The listing builds one solid part. Answer for the finished solid, in the listing's coordinates (mm). Face numbers are marked on the shaded views. A direction names the side the tool comes from. Round coordinates to 2 decimals unless told otherwise and drop trailing zeros. Loops run counter-clockwise (first coordinate to the right, second up) from the corner with the lowest first, then second, coordinate; pieces in that order, holes last. Notation, with made-up numbers: (-39.75, 51) - (-6.75, 51) arc R24 ccw to (-6.75, 71) - close; hole circle Ø3 at (34, 48). An arc over 180 degrees is marked (long way). One line per item, written item: value.
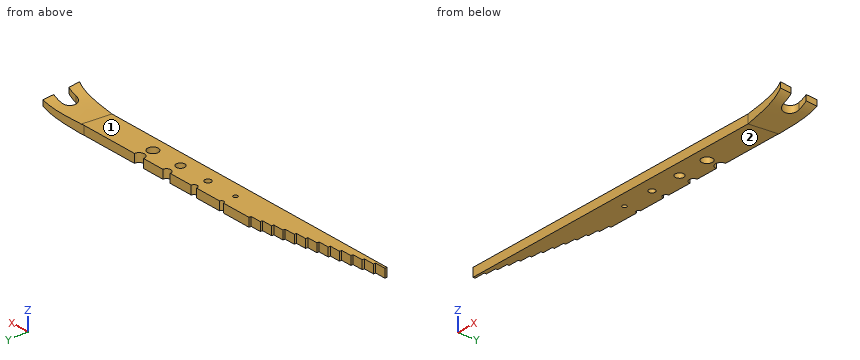
```python
from build123d import *

# Parameters (mm, degrees)
F0_R     = 1
F0_R_2   = 1.5
F0_R_3   = 2
F0_R_4   = 2.5
F1_DEPTH = 4
F3_DEPTH = 8
F5_DEPTH = 25


with BuildPart() as f1:
    # F0 (on Top) → F1 (new body)
    with BuildSketch(Plane.XY):
        with BuildLine():
            Line((-52.0707386732, -14.8954221606), (-52.0707386732, -15.8954221606))
            Line((-52.0707386732, -15.8954221606), (-57.0707386732, -15.8954221606))
            Line((-57.0707386732, -15.8954221606), (-57.0707386732, -16.8954221606))
            Line((-57.0707386732, -16.8954221606), (-62.0707386732, -16.8954221606))
            Line((-62.0707386732, -16.8954221606), (-62.0707386732, -17.8954221606))
            Line((-62.0707386732, -17.8954221606), (-67.0707386732, -17.8954221606))
            Line((-67.0707386732, -17.8954221606), (-67.0707386732, -18.8954221606))
            Line((-67.0707386732, -18.8954221606), (-72.0707386732, -18.8954221606))
            Line((-72.0707386732, -18.8954221606), (-72.0707386732, -19.8954221606))
            Line((-72.0707386732, -19.8954221606), (-77.0707386732, -19.8954221606))
            Line((-77.0707386732, -19.8954221606), (-77.0707386732, -20.8954221606))
            Line((-77.0707386732, -20.8954221606), (-82.0707386732, -20.8954221606))
            Line((-82.0707386732, -20.8954221606), (-82.0707386732, -21.8954221606))
            Line((-82.0707386732, -21.8954221606), (-87.0707386732, -21.8954221606))
            Line((-87.0707386732, -21.8954221606), (-87.0707386732, -22.8954221606))
            Line((-87.0707386732, -22.8954221606), (-92.0707386732, -22.8954221606))
            Line((-92.0707386732, -22.8954221606), (-92.0707386732, -23.8954221606))
            Line((-92.0707386732, -23.8954221606), (-97.0707386732, -23.8954221606))
            Line((-97.0707386732, -23.8954221606), (-97.0707386732, -24.8954221606))
            Line((-97.0707386732, -24.8954221606), (-102.0707386732, -24.8954221606))
            Line((-102.0707386732, -24.8954221606), (-102.0707386732, -25.8954221606))
            Line((-102.0707386732, -25.8954221606), (47.9292613268, -25.8954221606))
            Line((47.9292613268, -25.8954221606), (47.9292613268, -12.8954221606))
            Line((47.9292613268, -12.8954221606), (20.4292613268, -12.8954221606))
            ThreePointArc((20.4292613268, -12.8954221606), (17.9292613268, -15.3954221606), (15.4292613268, -12.8954221606))
            Line((15.4292613268, -12.8954221606), (4.9292613268, -12.8954221606))
            ThreePointArc((4.9292613268, -12.8954221606), (2.9292613268, -14.8954221606), (0.9292613268, -12.8954221606))
            Line((0.9292613268, -12.8954221606), (-10.5707386732, -12.8954221606))
            ThreePointArc((-10.5707386732, -12.8954221606), (-12.0707386732, -14.3954221606), (-13.5707386732, -12.8954221606))
            Line((-13.5707386732, -12.8954221606), (-26.0707386732, -12.8954221606))
            ThreePointArc((-26.0707386732, -12.8954221606), (-27.0707386732, -13.8954221606), (-28.0707386732, -12.8954221606))
            Line((-28.0707386732, -12.8954221606), (-42.0707386732, -12.8954221606))
            Line((-42.0707386732, -12.8954221606), (-42.0707386732, -13.8954221606))
            Line((-42.0707386732, -13.8954221606), (-47.0707386732, -13.8954221606))
            Line((-47.0707386732, -13.8954221606), (-47.0707386732, -14.8954221606))
            Line((-47.0707386732, -14.8954221606), (-52.0707386732, -14.8954221606))
        make_face()
        with Locations((-27.0707386732, -19.3954221606)):
            Circle(F0_R, mode=Mode.SUBTRACT)
        with Locations((-12.0707386732, -19.3954221606)):
            Circle(F0_R_2, mode=Mode.SUBTRACT)
        with Locations((2.9292613268, -19.3954221606)):
            Circle(F0_R_3, mode=Mode.SUBTRACT)
        with Locations((17.9292613268, -19.3954221606)):
            Circle(F0_R_4, mode=Mode.SUBTRACT)
    extrude(amount=F1_DEPTH)

    # F2 (on face) → F3 (join)
    with BuildSketch(Plane(origin=(0, 0, 0), x_dir=(1, 0, 0), z_dir=(0, 0, -1))):
        with BuildLine():
            Line((47.9292613268, 25.8954221606), (47.9292613268, 12.8954221606))
            Line((47.9292613268, 12.8954221606), (67.9292613268, 10.8954221606))
            Line((67.9292613268, 10.8954221606), (67.9292613268, 15.8954221606))
            Line((67.9292613268, 15.8954221606), (63.9292613268, 15.8954221606))
            ThreePointArc((63.9292613268, 15.8954221606), (60.4292613268, 19.3954221606), (63.9292613268, 22.8954221606))
            Line((63.9292613268, 22.8954221606), (67.9292613268, 22.8954221606))
            Line((67.9292613268, 22.8954221606), (67.9292613268, 27.8954221606))
            Line((67.9292613268, 27.8954221606), (47.9292613268, 25.8954221606))
        make_face()
    extrude(amount=-F3_DEPTH)

    # F4 (on face) → F5 (cut)
    with BuildSketch(Plane(origin=(-2.0893560424, -20.8935604237, 0), x_dir=(0.9950371902, -0.099503719, 0), z_dir=(-0.099503719, -0.9950371902, 0))):
        with BuildLine():
            Line((47.7105565369, 4), (50.2680883301, 4))
            Line((50.2680883301, 4), (50.2680883301, 8))
            Line((50.2680883301, 8), (70.3678395723, 8))
            add(Edge.make_bspline(
                [(70.3678395723, 8), (72.5567347198, 10.1579266461), (72.4264311984, 13.587186432), (72.296127677, 17.0164462179)],
                knots=[0.598533387, 0.598533387, 0.598533387, 0.598533387, 1, 1, 1, 1], degree=3))
            add(Edge.make_bspline(
                [(70.3678395723, 5.5720340461), (72.8712183365, 8.3489220533), (72.5836730067, 12.6826841356), (72.296127677, 17.0164462179)],
                knots=[0.5727584581, 0.5727584581, 0.5727584581, 0.5727584581, 1, 1, 1, 1], degree=3))
            Line((70.3678395723, 5.5720340461), (70.3678395723, 0))
            Line((70.3678395723, 0), (50.2680883301, 0))
            Line((50.2680883301, 0), (50.2680883301, -3.928697668))
            Line((50.2680883301, -3.928697668), (74.866913259, -3.928697668))
            Line((74.866913259, -3.928697668), (74.866913259, 19.5322930813))
            Line((74.866913259, 19.5322930813), (50.2680883301, 19.5322930813))
            Line((50.2680883301, 19.5322930813), (47.7105565369, 19.5322930813))
            Line((47.7105565369, 19.5322930813), (47.7105565369, 4))
        make_face()
        with BuildLine():
            Line((50.2680883301, 8), (50.2680883301, 4))
            add(Edge.make_bspline(
                [(50.2680883301, 4), (58.6862880108, 4.3914090203), (67.1044876915, 4.7828180407), (70.3678395723, 8)],
                knots=[0, 0, 0, 0, 0.598533387, 0.598533387, 0.598533387, 0.598533387], degree=3))
            Line((70.3678395723, 8), (50.2680883301, 8))
        make_face()
        with BuildLine():
            add(Edge.make_bspline(
                [(50.2680883301, 0), (58.6399537153, 0.9246740387), (67.0118191006, 1.8493480774), (70.3678395723, 5.5720340461)],
                knots=[0, 0, 0, 0, 0.5727584581, 0.5727584581, 0.5727584581, 0.5727584581], degree=3))
            Line((50.2680883301, 0), (70.3678395723, 0))
            Line((70.3678395723, 0), (70.3678395723, 5.5720340461))
        make_face()
    extrude(amount=-F5_DEPTH, mode=Mode.SUBTRACT)


solid = f1.part
```
1) A cutting plane is placed at B-B on x = 36.5. Give the vertices of the cut face in (y, z).
Final values:
outline: (-25.9, 0) - (-12.9, 0) - (-12.9, 4) - (-25.9, 4) - close
2) For the marked faces 1 and 2, determine the directions among +Z, -Z, +X, -X, +Y, -Y from which every point of the face is accessible in a straight line to the end or side of a thin tool.
Final values:
face 1: +Z, -X, +Y, -Y
face 2: -Z, +X, -X, +Y, -Y
3) A cutting plane is placed at A-A on x = -74. Give the vertices of the cut face in (y, z), and give its area (3 significant figures).
Final values:
outline: (-25.9, 0) - (-19.9, 0) - (-19.9, 4) - (-25.9, 4) - close
area: 24.0 mm2
4) Consider L1, parallel to Y at x = -40, z = 3.5; L2, parallel to Z at x = -90.5, y = -24.25; L3, parallel to Y at x = 55.5, z = 2. Determine where each line is inside the solid, lowest interval first.
Final values:
L1: -25.9 to -12.9
L2: 0 to 4
L3: -26.65 to -12.14
5) Each of these flat-tipped pins is pushed along its axis until it touches: pin 1 Ø3 at (x, z) = (-58.5, 2.5) entering from +Y; pin 2 Ø2 at (x, z) = (-29, 5.5) entering from +Y; pin 3 Ø3 at (x, z) = (-49.5, 2) entering from +Y; pin 4 Ø2 at (x, z) = (-95, 2) entering from +Y. Where does it stop, or does it pass through?
Final values:
pin 1: y = -15.9
pin 2: through
pin 3: y = -14.9
pin 4: y = -23.9
